For this review, use the dimensioned drawing (mm, ordinates from the lowest corner) and the shaded views. A direction names the side the tool comes from. Round coordinates to 2 decimals unless told otherwise and drop trailing zeros. Order: outer loops, then holes, each group sorted by start corner. A loop starts at its lowest first (then second) coordinate and runs counter-clockwise, first axis right, second up. Notation, with made-up numbers: (-37, -27) - (1, -27) arc R19 cw to (1, -10) - close; hole circle Ø8 at (-22.75, 36.5). An arc over 180 degrees is marked (long way). Write item = value, one per line.
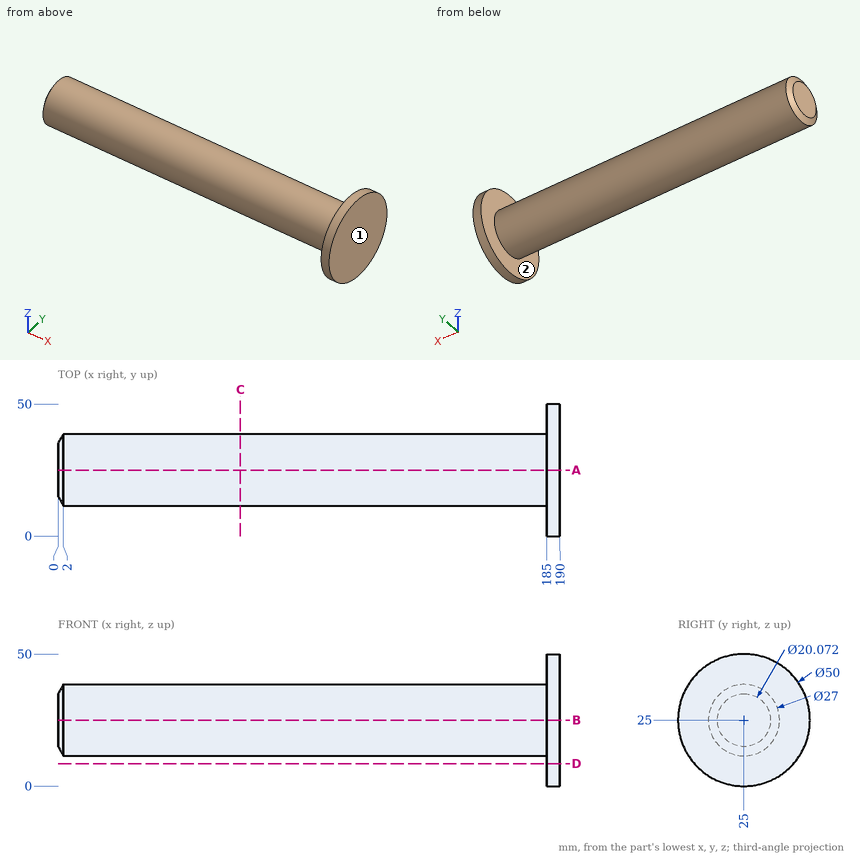
1) We need section A-A on y = 25. Write out the cut boundary in (x, z), and give its area (3 significant figures).
Findings:
outline = (0, 14.96) - (2, 11.5) - (185, 11.5) - (185, 0) - (190, 0) - (190, 50) - (185, 50) - (185, 38.5) - (2, 38.5) - (0, 35.04) - close
area = 5,240 mm^2
2) We need section D-D on z = 8.5. Write out the cut boundary in (x, y).
Findings:
outline = (185, 6.22) - (190, 6.22) - (190, 43.78) - (185, 43.78) - close
3) Clearance check with flat-ended pins moving along their axes: pin 1 Ø1.5 at (y, z) = (7, 26.5) entering from -X; pin 2 Ø10 at (x, y) = (107.5, 35) entering from -Z; pin 3 Ø12 at (x, z) = (124.5, 20) entering from +Y. State where each tip first meets the part, or that it passes through.
Findings:
pin_1 = 185
pin_2 = 12.46
pin_3 = 38.5
4) We need section C-C on x = 69. Write out the cut boundary in (y, z).
Findings:
outline = circle Ø27 at (25, 25)
5) For the marked faces 1 and 2, list the 3-axis set-ups (+Z, -Z, +X, -X, +Y, -Y) from which the entire face can be reached by the end or side of a thin tool; tool diameter is ignored.
Findings:
face_1 = +Z, -Z, +X, +Y, -Y
face_2 = -X
6) To check wall thickness, follow L1, parallel to Z at x = 55, y = 25.5; L2, parallel to X at y = 19, z = 40.5; L3, parallel to Z at x = 142, y = 16. State the ranges of each line that lie inside material, in increasing order. Write a range as from..to.
Findings:
L1 = 11.51..38.49
L2 = 185..190
L3 = 14.94..35.06
